```python
from build123d import *

# Parameters (mm, degrees)
SKETCH1_W                                      = 25.4
SKETCH1_H                                      = 12.7
BOSS_EXTRUDE1_DEPTH                            = 12.7
CBORE_FOR_8_SOCKET_HEAD_CAP_SCREW1_D           = 4.9149
CBORE_FOR_8_SOCKET_HEAD_CAP_SCREW1_CBORE_D     = 7.9375
CBORE_FOR_8_SOCKET_HEAD_CAP_SCREW1_CBORE_DEPTH = 5.08
M4X0_7_TAPPED_HOLE1_D                          = 3.3
M4X0_7_TAPPED_HOLE1_DEPTH                      = 11.6332
M4X0_7_TAPPED_HOLE1_TIP                        = 0.991420021


with BuildPart() as part:
    # Sketch1 → Boss-Extrude1 (new, symmetric)
    with BuildSketch(Plane.XY):
        Rectangle(SKETCH1_W, SKETCH1_H)
    extrude(amount=BOSS_EXTRUDE1_DEPTH, both=True)

    # CBORE for #8 Socket Head Cap Screw1 (through all)
    with Locations(Plane.XY.offset(12.7)):
        with Locations((-6.35, 0), (6.35, 0)):
            CounterBoreHole(CBORE_FOR_8_SOCKET_HEAD_CAP_SCREW1_D / 2, CBORE_FOR_8_SOCKET_HEAD_CAP_SCREW1_CBORE_D / 2, CBORE_FOR_8_SOCKET_HEAD_CAP_SCREW1_CBORE_DEPTH)

    # M4x0.7 Tapped Hole1
    with Locations(Plane(origin=(0, 6.35, 0), x_dir=(1, 0, 0), z_dir=(0, 1, 0))):
        with Locations((0, 0)):
            Hole(M4X0_7_TAPPED_HOLE1_D / 2, depth=M4X0_7_TAPPED_HOLE1_DEPTH)
            with Locations((0, 0, -(M4X0_7_TAPPED_HOLE1_DEPTH + M4X0_7_TAPPED_HOLE1_TIP / 2))):  # 118° drill point
                Cone(0, M4X0_7_TAPPED_HOLE1_D / 2, M4X0_7_TAPPED_HOLE1_TIP, mode=Mode.SUBTRACT)


solid = part.part
```
Verification items for the finished model (mm, model axes). A direction names the side the tool comes from. Give positions to 0.01 mm unless a question says otherwise; leave off trailing zeros. Loops run counter-clockwise (first coordinate to the right, second up) from the corner with the lowest first, then second, coordinate; pieces in that order, holes last. Notation, with made-up numbers: M 71,71.25 L 79,71.25 A8 ccw 79,86.25 Z; hole C -1,3 d2. An arc over 180 degrees is marked long. Return JSON: item names as keys, results as strings.
1) Material ranges on L1, parallel to Z at x = 0, y = 3; L2, parallel to Y at x = 6.35, z = 9.9; L3, parallel to X at y = -2.5, z = 7.75, recorded low to high. Write a range as [from, to].
Findings:
{"L1": "z = [-12.7, -1.65], [1.65, 12.7]", "L2": "y = [-6.35, -3.97], [3.97, 6.35]", "L3": "x = [-12.7, -9.43], [-3.27, 3.27], [9.43, 12.7]"}
2) Section check A-A, the plane y = 0. Enter the section's corners in (x, z), and give its area (3 significant figures).
Findings:
{"outline": "M -12.7,-12.7 L -8.81,-12.7 L -8.81,7.62 L -10.32,7.62 L -10.32,12.7 L -12.7,12.7 Z; M -3.89,-12.7 L 3.89,-12.7 L 3.89,7.62 L 2.38,7.62 L 2.38,12.7 L -2.38,12.7 L -2.38,7.62 L -3.89,7.62 Z; M 8.81,-12.7 L 12.7,-12.7 L 12.7,12.7 L 10.32,12.7 L 10.32,7.62 L 8.81,7.62 Z; hole C 0,0 d3.3", "area": "356 mm2"}
3) Section check D-D, the plane x = -4.25. Enter the section's corners in (y, z), and give its area (3 significant figures).
Findings:
{"outline": "M -6.35,-12.7 L -1.28,-12.7 L -1.28,7.62 L -3.37,7.62 L -3.37,12.7 L -6.35,12.7 Z; M 1.28,-12.7 L 6.35,-12.7 L 6.35,12.7 L 3.37,12.7 L 3.37,7.62 L 1.28,7.62 Z", "area": "236 mm2"}
4) Section check B-B, the plane x = 6.35. Enter the section's corners in (y, z), and give its area (3 significant figures).
Findings:
{"outline": "M -6.35,-12.7 L -2.46,-12.7 L -2.46,7.62 L -3.97,7.62 L -3.97,12.7 L -6.35,12.7 Z; M 2.46,-12.7 L 6.35,-12.7 L 6.35,12.7 L 3.97,12.7 L 3.97,7.62 L 2.46,7.62 Z", "area": "182 mm2"}
5) Gauge pin test, flat ends, axial feed: P1, Ø3, axis at x = 8, y = -2.5, coming from the +Z side; P2, Ø2, axis at x = 0, z = 0, coming from the +Y side; P3, Ø3, axis at x = -7.5, y = -1, coming from the +Z side; P4, Ø3, axis at x = 6.35, y = 0, coming from the -Z side. Record the tip position at first contact, or that the pin passes through.
Findings:
{"P1": "stops at z = 12.7", "P2": "stops at y = -5.67", "P3": "stops at z = 7.62", "P4": "passes through"}
6) Tool access check on faces 5 (the cylindrical face through (10.135, 1.192, 10.196)), 6 (the cylindrical face through (-3.895, 0.108, -2.682)). Record the directions out of +Z, -Z, +X, -X, +Y, -Y that give a thin tool (end or side, any length) a straight path to the whole face; none if there is none.
Findings:
{"face 5": "+Z", "face 6": "+Z, -Z"}
7) Mould release check, pull along Z, two halves, no side actions. Record for faces 1 (the cylindrical face through (4.08, -0.94, -2.68)), 2 (the flat face through (0, 0, -12.7)), 3 (the cylindrical face through (1.216, 0.452, -1.115)), 4 (the flat face through (9, 0, 7.62)): released by +Z, released by -Z, zero draft, split by the parting line, or undercut.
Findings:
{"face 1": "zero draft", "face 2": "released by -Z", "face 3": "undercut", "face 4": "released by +Z"}
8) Section check C-C, the plane z = 4.5. Enter the section's corners in (x, y), and give its area (3 significant figures).
Findings:
{"outline": "M -12.7,-6.35 L 12.7,-6.35 L 12.7,6.35 L -12.7,6.35 Z; hole C -6.35,0 d4.91; hole C 6.35,0 d4.91", "area": "285 mm2"}
